For this review, take the finished solid that the model builds, in its own axes (mm). Face numbers are marked on the shaded views. A direction names the side the tool comes from. Coordinates: 2 decimals unless noted, no trailing zeros. Write item = value, one per line. Start each with the question number.
1) Machinability: for the marked faces 4, 5 and 6, which of the approach directions +Z, -Z, +X, -X, +Y, -Y give a long, thin tool a straight path to every point of the face, cutting with its end or side? Answer none if there is none.
2) Insertion check: pin 1 Ø10 at (y, z) = (-74, 160.5) entering from -X; pin 2 Ø3 at (y, z) = (-69, -46.5) entering from +X; pin 3 Ø3 at (y, z) = (-59.5, -132) entering from -X; pin 4 Ø13.5 at (x, z) = (-60, -103.92) entering from +Y. Each pin has a flat end and moves straight along its axis. Give the tip position at first contact, or say it passes through.
3) Draft analysis for pull direction X (two halves, no side actions). For the marked faces 1, 2 and 3, state which applies: +X half, -X half, draft (parallel to the pull), parting line (faces both ways), or undercut.
4) Wall thickness on probe 1 along Z at (x, y) = (-5, -79); probe 2 along Z at (x, y) = (-68.5, -23.5); probe 3 along Y at (x, z) = (161.5, 128): over which ranges is each line inside the solid? List them lowest first. Write a range as [from, to].
from build123d import *

# Parameters (mm, degrees)
CUT_EXTRUDE_1_DEPTH      = 15
SKETCH_3_R               = 4.25
CUT_EXTRUDE_2_DEPTH      = 20
PATTERN_CIRCULAR_1_COUNT = 6
CUT_EXTRUDE_3_REACH      = 337.203
SKETCH_4_R               = 6.5
PATTERN_CIRCULAR_2_COUNT = 6
SKETCH_5_R               = 4.25
CUT_EXTRUDE_4_DEPTH      = 20
CUT_EXTRUDE_5_REACH      = 453.217
SKETCH_6_R               = 4


with BuildPart() as part:
    # 草图1 → 旋转1 (revolve)
    with BuildSketch(Plane.XY, mode=Mode.PRIVATE) as revolve_1_sk:
        Polygon((-150, 0), (-100, 0), (-100, -16), (-86.5, -16), (-86.5, -24), (-170, -24), (-190, -44), (-190, -54.5), (-180, -54.5), (-180, -76), (-195, -76), (-195, -86), (-200, -86), (-200, -34), (-230, -34), (-230, -5), (-150, -5), align=None)
    revolve(revolve_1_sk.sketch.rotate(Axis((0, 0, 0), (0, -1, 0)), 270), axis=Axis((0, 0, 0), (0, -1, 0)))

    # 草图2 → 切除-拉伸1 (cut, symmetric)
    with BuildSketch(Plane.XY):
        Polygon((201.17641936, -5), (222.039301067, -29), (230, -29), (230, -5), align=None)
    extrude(amount=CUT_EXTRUDE_1_DEPTH, both=True, mode=Mode.SUBTRACT)

    # 草图3 → 切除-拉伸2 (cut)
    with BuildSketch(Plane(origin=(0, 0, 0), x_dir=(1, 0, 0), z_dir=(0, 1, 0))):
        with Locations(Location((120, 0, 0), (0, 0, 270))):
            Circle(SKETCH_3_R)
    cut_extrude_2 = extrude(amount=-CUT_EXTRUDE_2_DEPTH, mode=Mode.SUBTRACT)

    # 阵列(圆周)1: 切除-拉伸2 ×6 about axis
    pattern_circular_1_axis = Axis((0, 0, 0), (0, 1, 0))
    for i in range(1, PATTERN_CIRCULAR_1_COUNT):
        add(cut_extrude_2.rotate(pattern_circular_1_axis, i * 360 / PATTERN_CIRCULAR_1_COUNT), mode=Mode.SUBTRACT)

    # 草图4 → 切除-拉伸3 (cut, up to next)
    with BuildSketch(Plane(origin=(0, -5, 0), x_dir=(1, 0, 0), z_dir=(0, 1, 0)), mode=Mode.PRIVATE) as cut_extrude_3_sk1:
        with Locations(Location((55.646094697, -207.674052652, 0), (0, 0, 270))):
            Circle(SKETCH_4_R)
    cut_extrude_3_tool1 = extrude(cut_extrude_3_sk1.sketch, amount=-CUT_EXTRUDE_3_REACH, mode=Mode.PRIVATE) & part.part
    cut_extrude_3 = cut_extrude_3_tool1.solids().sort_by_distance((55.646095, -5, 207.674053))[0]
    add(cut_extrude_3, mode=Mode.SUBTRACT)

    # 阵列(圆周)2: 切除-拉伸3 ×6 about axis
    pattern_circular_2_axis = Axis((0, 0, 0), (0, 1, 0))
    for i in range(1, PATTERN_CIRCULAR_2_COUNT):
        add(cut_extrude_3.rotate(pattern_circular_2_axis, i * 360 / PATTERN_CIRCULAR_2_COUNT), mode=Mode.SUBTRACT)

    # 草图5 → 切除-拉伸4 (cut)
    with BuildSketch(Plane(origin=(112.111712569, 97.45722489, 0), x_dir=(0, 0, -1), z_dir=(0.7547095802227705, 0.656059028990509, 0))):
        with Locations(Location((0, -147.682271182, 0), (0, 0, 90))):
            Circle(SKETCH_5_R)
    extrude(amount=-CUT_EXTRUDE_4_DEPTH, mode=Mode.SUBTRACT)

    # 切除-拉伸5: up to this cone (the profile starts outside it)
    cut_extrude_5_end = Plane(origin=(0, -14, 0), z_dir=(0, -1, 0)).offset(-159.999999) * Cone(1e-06, 773.717, 773.716999, align=(Align.CENTER, Align.CENTER, Align.MIN), mode=Mode.PRIVATE)
    # 草图6 → 切除-拉伸5 (cut, up to the surface)
    with BuildSketch(Plane(origin=(112.111712569, 97.45722489, 0), x_dir=(0, 0, -1), z_dir=(0.7547095802227705, 0.656059028990509, 0)), mode=Mode.PRIVATE) as cut_extrude_5_sk1:
        with Locations(Location((0, -147.682271182, 0), (0, 0, 90))):
            Circle(SKETCH_6_R)
    cut_extrude_5_tool1 = extrude(cut_extrude_5_sk1.sketch, amount=-CUT_EXTRUDE_5_REACH, mode=Mode.PRIVATE) - cut_extrude_5_end
    add(cut_extrude_5_tool1.solids().sort_by_distance((209, -14, 0))[0], mode=Mode.SUBTRACT)


solid = part.part
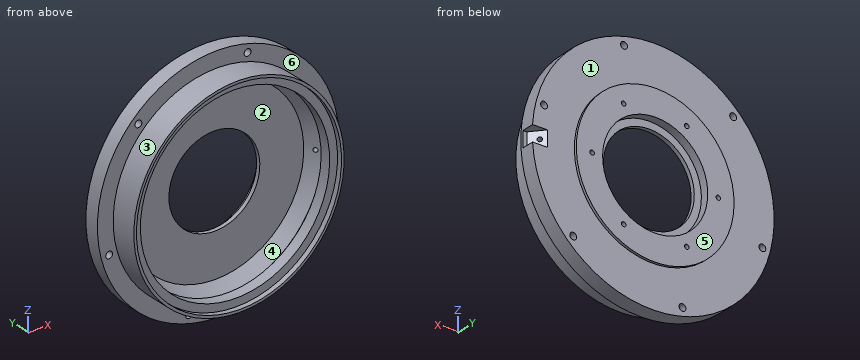
Answer sheet:
q1.face_4 = none
q1.face_5 = +Z, -Z, +X, -X, +Y
q1.face_6 = -Y
q2.pin_1 = -125.78
q2.pin_2 = 194.87
q2.pin_3 = -151.56
q2.pin_4 = 0
q3.face_1 = draft
q3.face_2 = undercut
q3.face_3 = parting line
q4.probe_1 = [-199.94, -194.94], [194.94, 199.94]
q4.probe_2 = [-219.56, -52.82], [52.82, 219.56]
q4.probe_3 = [-34, -5]
